Autodesk Inventor part; units mm, degrees
ref_plane "YZ Plane" through (0, 0, 0) normal (1, 0, 0) x (0, 1, 0)
ref_plane "XZ Plane" through (0, 0, 0) normal (0, 1, 0) x (-1, 0, 0)
ref_plane "XY Plane" through (0, 0, 0) normal (0, 0, 1) x (1, 0, 0)
sketch "Sketch1" plane through (0, 0, 0) normal (1, 0, 0) x (0, 1, 0)
  circle A0 centre (0, 0) radius 4
  dimension "d0" = 8
extrude "Extrusion1" add sketch "Sketch1" along normal blind 80
sketch "Sketch8" plane through (80, 0, 0) normal (1, 0, 0) x (0, 0, -1)
  line L0 (-10, -3.7509) -> (-10, 5.6543)
  circle A0 centre (0, 0) radius 4
  point P0 (-10, 0.9517)
  dimension "d13" = 10
revolve "Revolution2" add sketch "Sketch8" angle 90 about axis through (80, -3.7509, 10) along (0, -1, 0)
sketch "Sketch9" plane through (90, 0, 10) normal (0, 0, 1) x (1, 0, 0)
  circle A0 centre (0, 0) radius 4
  point P0 (-90, 0)
extrude "Extrusion6" add sketch "Sketch9" along normal blind 20
sketch "Sketch10" plane through (0, 0, 0) normal (-1, 0, 0) x (0, 0, 1)
  circle A0 centre (0, 0) radius 4
  line L0 (0, -4.7151) -> (0, 4)
  point P0 (0, -4)
extrude "Extrusion7" cut sketch "Sketch10" against normal blind 20 contours A0 L0 picked at (0.5785, 1.2013)
properties part number "AllenKey-RS3" material "Steel"
Could you check a few things on this model? Use its own coordinates, in mm. A direction names the side the tool comes from. Coordinates: 2 decimals unless noted, no trailing zeros. Loops run counter-clockwise (first coordinate to the right, second up) from the corner with the lowest first, then second, coordinate; pieces in that order, holes last.
1. I need wall thicknesses on L1, parallel to Z at x = 28.5, y = 0; L2, parallel to X at y = 0.25, z = 18; L3, parallel to X at y = -2.5, z = 11.5. Which ranges of each line are inside material? Lowest first, please.
2. Imagine slicing it at B-B (x = 9). Please give me the cut outline in (y, z), and give its area (3 significant figures).
3. For faces 1 (the face through (90, 0, 30)), 2 (the face through (86, 0, 20)), 3 (the face through (20, 0, 2)), 4 (the face through (39.44, -0.521, -3.966)), which set-ups out of +Z, -Z, +X, -X, +Y, -Y let a thin tool reach every point of the face, with its end or its side?
4. Imagine slicing it at C-C (z = 13). Please give me the cut outline in (x, y), and give its area (3 significant figures).
5. Imagine slicing it at D-D (x = 58.5). Please give me the cut outline in (y, z), and give its area (3 significant figures).
6. For P1, Ø2, axis at y = -2.5, z = 20.5, coming from the +X side; P2, Ø3, axis at y = -3, z = 1.5, coming from the +X side, each with a flat end and sliding along its axis, tell me the tip position at first contact or that it passes through.
7. Imagine slicing it at A-A (y = 0). Please give me the cut outline in (x, z), and give its area (3 significant figures).
Computed values:
1. L1: z = -4 to 4
1. L2: x = 86.01 to 93.99
1. L3: x = 86.88 to 93.12
2. outline: (-4, 0) arc R4 ccw to (4, 0) - close
2. area: 25.1 mm2
3. face 1: +Z, +X, -X, +Y, -Y
3. face 2: +Z
3. face 3: +Z, -X, +Y, -Y
3. face 4: -X
4. outline: circle Ø8 at (90, 0)
4. area: 50.3 mm2
5. outline: circle Ø8 at (0, 0)
5. area: 50.3 mm2
6. P1: stops at x = 93.71
6. P2: stops at x = 91.26
7. outline: (0, -4) - (80, -4) arc R14 ccw to (94, 10) - (94, 30) - (86, 30) - (86, 10) arc R6 cw to (80, 4) - (20, 4) - (20, 0) - (0, 0) - close
7. area: 846 mm2
